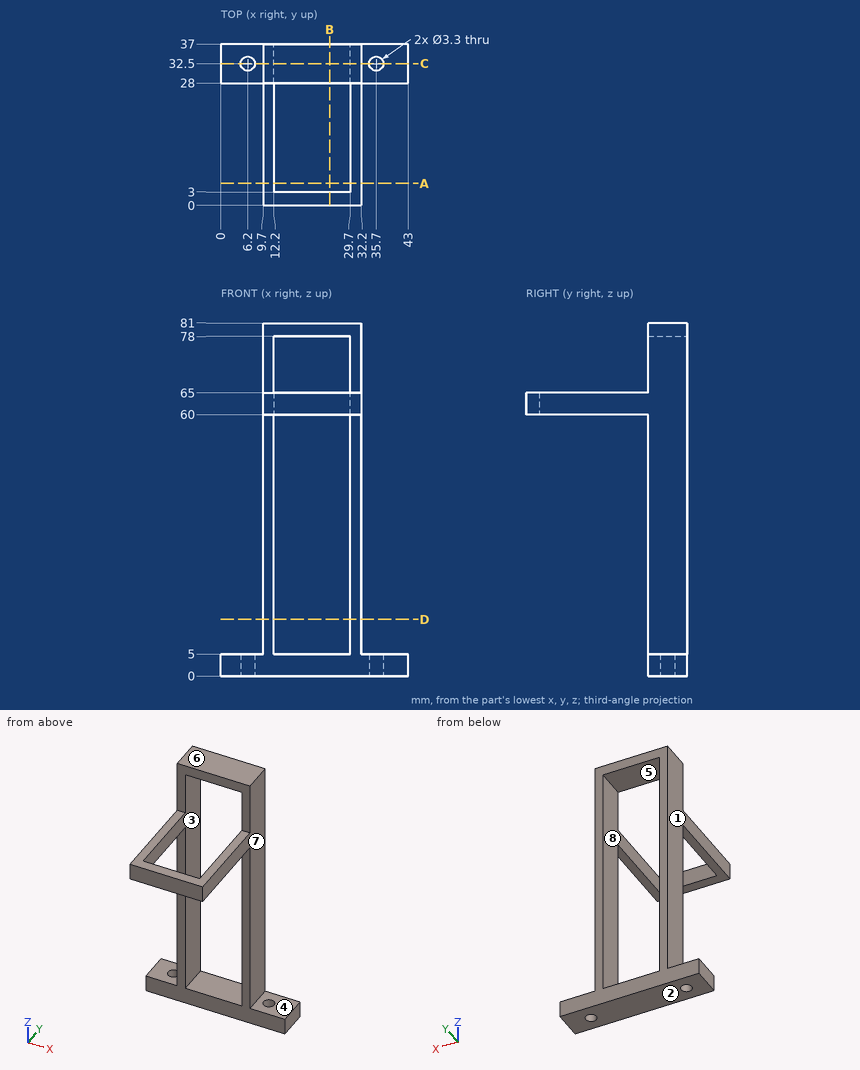
Could you check a few things on this drawing? It's one solid part, dimensions in mm from its lowest x, y, z. A direction names the side the tool comes from. Coordinates: 2 decimals unless noted, no trailing zeros. Write each loop counter-clockwise with the first axis right and the second up, starting at its lowest first coordinate (ties: lowest second). Pieces come first, ordered by that corner, then holes.
Q1. Imagine slicing it at A-A, the plane y = 5. List the corners of the cut face in (x, z) for me, plus the area to 3 significant figures.
Results found:
outline: (9.7, 60) - (12.2, 60) - (12.2, 65) - (9.7, 65) - close; (29.7, 60) - (32.2, 60) - (32.2, 65) - (29.7, 65) - close
area: 25.0 mm2
Q2. Please list where these lines run through material, in increasing order: L1, parallel to X at y = 32.5, z = 3.7; L2, parallel to Y at x = 35.7, z = 4.05; L3, parallel to X at y = 31.5, z = 52.
Results found:
L1: x = 0 to 4.55, 7.85 to 34.05, 37.35 to 43
L2: y = 28 to 30.85, 34.15 to 37
L3: x = 9.7 to 12.2, 29.7 to 32.2
Q3. If we mould it in two halves opening along Z, with no side actions, what happens to the marked faces 1, 2, 3 and 4? For each: +Z half, -Z half, draft (parallel to the pull), parting line (faces both ways), or undercut.
Results found:
face 1: draft
face 2: -Z half
face 3: undercut
face 4: +Z half
Q4. Imagine slicing it at C-C, the plane y = 32.5. List the corners of the cut face in (x, z) for me, plus the area to 4 significant figures.
Results found:
outline: (0, 0) - (4.55, 0) - (4.55, 5) - (0, 5) - close; (7.85, 0) - (34.05, 0) - (34.05, 5) - (32.2, 5) - (32.2, 81) - (9.7, 81) - (9.7, 5) - (7.85, 5) - close; (37.35, 0) - (43, 0) - (43, 5) - (37.35, 5) - close; hole (12.2, 5) - (29.7, 5) - (29.7, 78) - (12.2, 78) - close
area: 614.5 mm2
Q5. Imagine slicing it at D-D, the plane z = 13. List the corners of the cut face in (x, y) for me.
Results found:
outline: (9.7, 28) - (12.2, 28) - (12.2, 37) - (9.7, 37) - close; (29.7, 28) - (32.2, 28) - (32.2, 37) - (29.7, 37) - close
Q6. Which directions (+Z, -Z, +X, -X, +Y, -Y) give clear straight access to the entire face, cutting with the end or side of a thin tool? Please do the marked faces 5, 6, 7 and 8.
Results found:
face 5: +Y, -Y
face 6: +Z, +X, -X, +Y, -Y
face 7: +Z, +X, +Y, -Y
face 8: +Y
Q7. Imagine slicing it at B-B, the plane x = 25. List the corners of the cut face in (y, z) for me.
Results found:
outline: (0, 60) - (3, 60) - (3, 65) - (0, 65) - close; (28, 0) - (37, 0) - (37, 5) - (28, 5) - close; (28, 78) - (37, 78) - (37, 81) - (28, 81) - close
Q8. For P1, Ø4.5, axis at x = 6, y = 30.5, coming from the +Z side; P2, Ø2, axis at x = 12, y = 14, coming from the +Z side; P3, Ø5.5, axis at x = 6.2, y = 32.5, coming from the -Z side; P4, Ø1.5, axis at x = 21, z = 63.5, coming from the +Y side, each with a flat end and sliding along its axis, tell me the tip position at first contact or that it passes through.
Results found:
P1: stops at z = 5
P2: stops at z = 65
P3: stops at z = 0
P4: stops at y = 3
